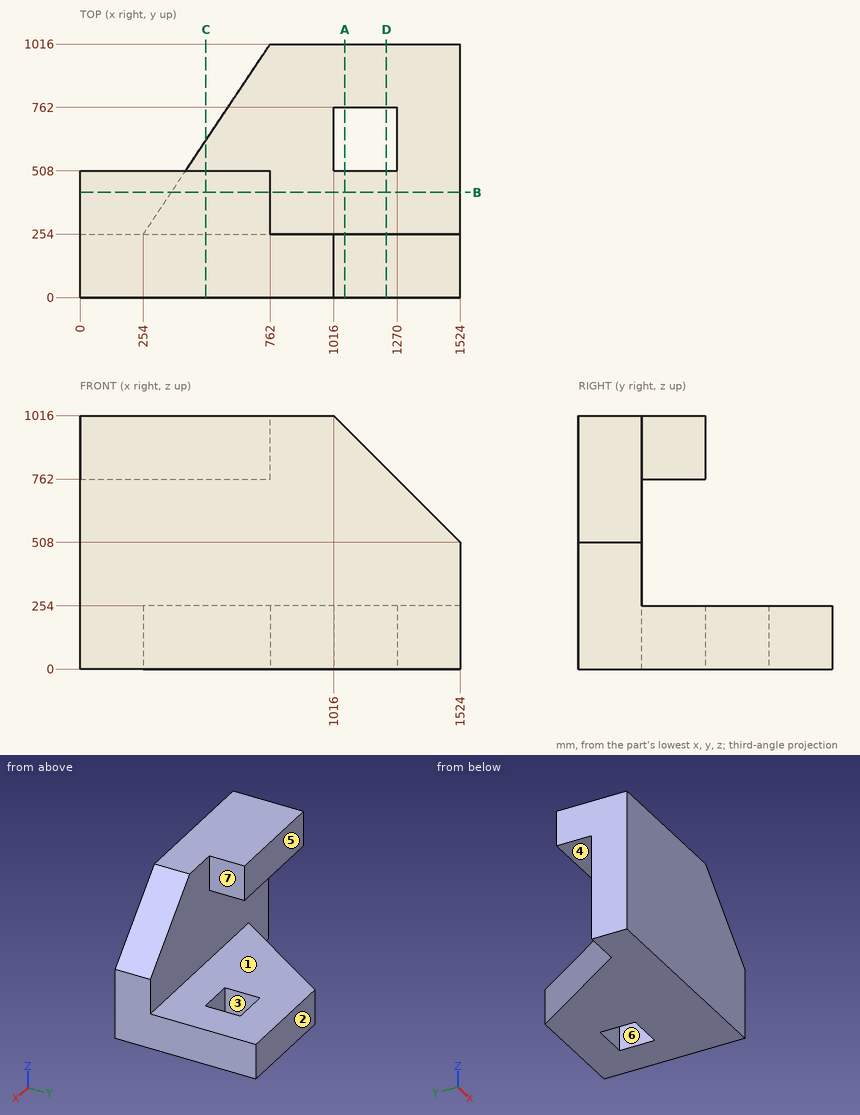
Can you work these out from the drawing? Everything is in mm from the part's minimum corner. A direction names the side the tool comes from. Give positions to 0.01 mm unless a question says otherwise; leave off trailing zeros. Order: outer loops, then holes, each group sorted by start corner. A loop starts at its lowest first (then second) coordinate and runs counter-clockwise, first axis right, second up.
1. I need wall thicknesses on L1, parallel to Z at x = 643.5, y = 427; L2, parallel to Y at x = 1207, z = 92.5; L3, parallel to X at y = 387.5, z = 922. Which ranges of each line are inside material? Lowest first, please.
2. Will these pins go through, and if not, where does the flat tip stop? P1, Ø5, axis at x = 761, y = 538, coming from the +Z side; P2, Ø5, axis at y = 616.5, z = 109.5, coming from the -X side.
3. Suppose I cut it at D-D (x = 1227). List the corners of the cut face in (y, z) for me, plus the area to 3 significant figures.
4. We'd pull the mould along Y, two halves only. Please class the marked faces 1, 2 and 3: pulls with the +Y half, pulls with the -Y half, needs draft (parallel to the pull), parting line crosses it, or undercut.
5. Suppose I cut it at B-B (y = 422). List the corners of the cut face in (x, z) for me.
6. Suppose I cut it at A-A (x = 1061). List the corners of the cut face in (y, z) for me.
7. Suppose I cut it at C-C (x = 504.5). List the corners of the cut face in (y, z) for me.
8. For the marked faces 4, 5, 6 and 7, which set-ups out of +Z, -Z, +X, -X, +Y, -Y let a thin tool reach every point of the face, with its end or its side?
Solved:
1. L1: z = 0 to 254, 762 to 1016
1. L2: y = 0 to 508, 762 to 1016
1. L3: x = 0 to 762
2. P1: stops at z = 254
2. P2: stops at x = 494
3. outline: (0, 0) - (508, 0) - (508, 254) - (254, 254) - (254, 805) - (0, 805) - close; (762, 0) - (1016, 0) - (1016, 254) - (762, 254) - close
3. area: 334,000 mm2
4. face 1: needs draft
4. face 2: pulls with the +Y half
4. face 3: undercut
5. outline: (0, 762) - (762, 762) - (762, 1016) - (0, 1016) - close; (366, 0) - (1524, 0) - (1524, 254) - (366, 254) - close
6. outline: (0, 0) - (508, 0) - (508, 254) - (254, 254) - (254, 971) - (0, 971) - close; (762, 0) - (1016, 0) - (1016, 254) - (762, 254) - close
7. outline: (0, 0) - (629.75, 0) - (629.75, 254) - (254, 254) - (254, 762) - (508, 762) - (508, 1016) - (0, 1016) - close
8. face 4: +X, -X, +Y
8. face 5: +Z, +X, -X, +Y
8. face 6: +Z, -Z
8. face 7: +Z, +X, +Y
